```python
from build123d import *

# Parameters (mm, degrees)
BOSS_EXTRU_1_DEPTH           = 5.2
BOSS_EXTRU_2_DEPTH           = 2
R_P_TITION_CIRCULAIRE1_COUNT = 10
ESQUISSE2_W                  = 6.2
ESQUISSE2_H                  = 6.2
ENL_V_MAT_EXTRU_1_DEPTH      = 8.2


with BuildPart() as part:
    # Esquisse1 → Boss.-Extru.1 (new body)
    with BuildSketch(Plane.XY):
        with BuildLine():
            Line((-5, 15.388417686), (0, 0))
            Line((0, 0), (5, 15.388417686))
            ThreePointArc((5, 15.388417686), (3.491302077, 15.799183798), (1.95, 16.062406385))
            Line((1.95, 16.062406385), (1.875, 19.061468738))
            Line((1.875, 19.061468738), (-1.875, 19.061468738))
            Line((-1.875, 19.061468738), (-1.95, 16.062406385))
            ThreePointArc((-1.95, 16.062406385), (-3.491302077, 15.799183798), (-5, 15.388417686))
        make_face()
    boss_extru_1 = extrude(amount=BOSS_EXTRU_1_DEPTH)

    # Esquisse4 → Boss.-Extru.2 (add)
    with BuildSketch(Plane(origin=(0, 0, 0), x_dir=(-1, 0, 0), z_dir=(0, 0, -1))):
        Polygon((0, 0), (-6.193446632, 19.061468738), (6.193446632, 19.061468738), align=None)
    boss_extru_2 = extrude(amount=BOSS_EXTRU_2_DEPTH)

    # Répétition circulaire1: Boss.-Extru.1, Boss.-Extru.2 ×10 about axis
    r_p_tition_circulaire1_axis = Axis((0, 0, 0), (0, 0, 1))
    for i in range(1, R_P_TITION_CIRCULAIRE1_COUNT):
        add(boss_extru_1.rotate(r_p_tition_circulaire1_axis, i * 360 / R_P_TITION_CIRCULAIRE1_COUNT))
        add(boss_extru_2.rotate(r_p_tition_circulaire1_axis, i * 360 / R_P_TITION_CIRCULAIRE1_COUNT))

    # Esquisse2 → Enlèv. mat.-Extru.1 (cut, through all)
    with BuildSketch(Plane.XY.offset(5.2)):
        Rectangle(ESQUISSE2_W, ESQUISSE2_H)
    extrude(amount=-ENL_V_MAT_EXTRU_1_DEPTH, mode=Mode.SUBTRACT)


solid = part.part
```
Work out the finished part from the listing and answer in its coordinate system (mm). A direction names the side the tool comes from. Give positions to 0.01 mm unless a question says otherwise; leave off trailing zeros. Order: outer loops, then holes, each group sorted by start corner. A loop starts at its lowest first (then second) coordinate and runs counter-clockwise, first axis right, second up. Notation, with made-up numbers: (49, -21) - (82, -21) arc R30 cw to (82, 13) - close; hole circle Ø6 at (-8.75, 18.25). An arc over 180 degrees is marked (long way). One line per item, written item: value. Start each with the question number.
1. Each of these flat-tipped pins is pushed along its axis until it touches: pin 1 Ø2 at (x, y) = (-18, -1.5) entering from +Z; pin 2 Ø2 at (y, z) = (7.5, 0.5) entering from +X; pin 3 Ø2 at (y, z) = (13, 4) entering from -X. Where does it stop, or does it pass through?
2. Section B-B, the plane y = -2.5 is taken. Write down the section's boundary in (x, z).
3. For a pull along Y with two mould halves and no side action, classify faces 6 (the face through (0, -19.061, 1)), 7 (the face through (-17.27, -3.6, 2.56)), 8 (the face through (-8.763, 15.315, 2.564)), 9 (the face through (5, -17, 0)) as released by +Y, released by -Y, zero draft, split by the parting line, or undercut.
4. Section A-A, the plane z = -1.5 is taken. Write down the section's boundary in (x, y), then the cut area to 3 significant figures.
5. Consider line 1 (Y direction, x = 1.5, z = -1.25); line 2 (Y direction, x = -11.5, z = 1.5); line 3 (Z direction, x = 18.5, y = -4). Determine where each line is inside the solid, lowest interval first.
6. Section D-D, the plane y = -10 is taken. Write down the section's boundary in (x, z), then the cut area to 3 significant figures.
7. Section C-C, the plane x = -9 is taken. Write down the section's boundary in (y, z).
8. Which of the six approach directions +Z, -Z, +X, -X, +Y, -Y give full straight-line access (tool end or side, diameter ignored) to faces 1 (the face through (5, 17, 0)), 2 (the face through (16.09, -7.24, 2.56)), 3 (the face through (11.134, -15.472, 0.85)), 4 (the face through (-18, 0, 0)), 5 (the face through (17.27, 3.6, 2.56))?
Filled sheet:
1. pin 1: z = 0
1. pin 2: x = 17.93
1. pin 3: x = -12.5
2. outline: (-19.23, -2) - (-3.1, -2) - (-3.1, 5.2) - (-15.99, 5.2) - (-15.99, 0) - (-19.23, 0) - close; (3.1, -2) - (19.23, -2) - (19.23, 0) - (15.99, 0) - (15.99, 5.2) - (3.1, 5.2) - close
3. face 6: released by -Y
3. face 7: undercut
3. face 8: released by +Y
3. face 9: zero draft
4. outline: (-20.04, 0) - (-16.21, -11.78) - (-6.19, -19.06) - (6.19, -19.06) - (16.21, -11.78) - (20.04, 0) - (16.21, 11.78) - (6.19, 19.06) - (-6.19, 19.06) - (-16.21, 11.78) - close; hole (-3.1, -3.1) - (3.1, -3.1) - (3.1, 3.1) - (-3.1, 3.1) - close
4. area: 1,140 mm²
5. line 1: -19.06 to -3.1, 3.1 to 19.06
5. line 2: -15.21 to -12.55, -11.38 to 11.38, 12.55 to 15.21
5. line 3: -2 to 0
6. outline: (-16.79, -2) - (16.79, -2) - (16.79, 0) - (12.72, 0) - (12.72, 5.2) - (-12.72, 5.2) - (-12.72, 0) - (-16.79, 0) - close
6. area: 199 mm²
7. outline: (-17.02, -2) - (17.02, -2) - (17.02, 0) - (15.63, 0) - (15.63, 5.2) - (-15.63, 5.2) - (-15.63, 0) - (-17.02, 0) - close
8. face 1: +Z, +Y
8. face 2: +Z, -Y
8. face 3: +Z, -Z, +X, -Y
8. face 4: +Z, -X
8. face 5: +Z, +X
